Input: part model. Units: mm. Frame: model coordinates. A direction names the side the tool comes from. Round coordinates to 2 decimals unless told otherwise and drop trailing zeros. Loops run counter-clockwise (first coordinate to the right, second up) from the corner with the lowest first, then second, coordinate; pieces in that order, holes last.
1) First-contact query: pin 1 (3 mm diameter, centred on x = -9.5, y = 14, fed in from +Z); pin 2 (3 mm diameter, centred on x = -83.5, z = -66.5, fed in from -Y); pin 3 (4 mm diameter, centred on x = -109.51, z = 1.14, fed in from +Y). Flat tips, straight axial feed; report the tip coordinate or a pass-through.
2) Section B-B, the plane y = 12. Return loops of the section in (x, z) (3 decimals).
3) Section D-D, the plane x = -33.5. Return loops of the section in (y, z), and give its area (3 significant figures).
4) Section C-C, the plane z = -24. Return loops of the section in (x, y).
5) Section A-A, the plane y = 35.5. Return loops of the section in (x, z), and give its area (3 significant figures).
6) Ray query, line 1 along Z through (x, y) = (-47, 4); line 2 along X through (y, z) = (34.5, -31); line 3 along X through (y, z) = (33, -42.5). Return the intervals inside material, ascending.
7) Draft query along Z for faces 1 (the face through (-37.63, 34.53, -57.46)), 2 (the face through (-104.37, 18.68, -4.43)), 3 (the face through (-7, 32.675, -104)). Return one class per face: pulls with the +Z half, pulls with the -Z half, needs draft (parallel to the pull), parting line crosses it, or undercut.
8) Access query for faces 4 (the face through (-103.37, 3.13, -86.91)), 5 (the face through (-107, 32.675, 0)), 6 (the face through (-103.944, 18.682, -98.721)), 7 (the face through (-7, 32.675, -1)). Directions: +Z, -Z, +X, -X, +Y, -Y. A direction counts if a zero-diameter tool reaches every point of the face in a straight line with its end or side. Return the directions, or none.
from build123d import *

# Parameters (mm, degrees)
SKETCH1_W           = 119.38
SKETCH1_H           = 119.38
BOSS_EXTRUDE1_DEPTH = 37.75
SKETCH2_R           = 2.286
CUT_EXTRUDE1_DEPTH  = 38.75
SKETCH3_R           = 58.41973455
CUT_EXTRUDE2_DEPTH  = 6.35
SKETCH4_R           = 58.42
CUT_EXTRUDE3_DEPTH  = 6.35
SKETCH5_R           = 20.32
BOSS_EXTRUDE2_DEPTH = 6.35
SKETCH6_R           = 20.32
BOSS_EXTRUDE3_DEPTH = 6.35
FILLET1_R           = 5.08
SKETCH7_R           = 88.9
SKETCH7_R_2         = 66.675
CUT_EXTRUDE5_DEPTH  = 13.8


with BuildPart() as part:
    # Sketch1 → Boss-Extrude1 (new body)
    with BuildSketch(Plane(origin=(0, 0, 0), x_dir=(1, 0, 0), z_dir=(0, 1, 0))):
        with Locations((-57.011822664, 51.361162791)):
            Rectangle(SKETCH1_W, SKETCH1_H)
    extrude(amount=BOSS_EXTRUDE1_DEPTH)

    # Sketch2 → Cut-Extrude1 (cut, through all)
    with BuildSketch(Plane(origin=(0, 37.75, 0), x_dir=(1, 0, 0), z_dir=(0, 1, 0))):
        with Locations((-109.511822664, 103.861162791)):
            Circle(SKETCH2_R)
        with Locations((-4.511822664, 103.861162791)):
            Circle(SKETCH2_R)
        with Locations((-4.511822664, -1.138837209)):
            Circle(SKETCH2_R)
        with Locations((-109.511822664, -1.138837209)):
            Circle(SKETCH2_R)
    extrude(amount=-CUT_EXTRUDE1_DEPTH, mode=Mode.SUBTRACT)

    # Sketch3 → Cut-Extrude2 (cut)
    with BuildSketch(Plane(origin=(0, 37.75, 0), x_dir=(1, 0, 0), z_dir=(0, 1, 0))):
        with Locations((-57.011822664, 51.361162791)):
            Circle(SKETCH3_R)
    extrude(amount=-CUT_EXTRUDE2_DEPTH, mode=Mode.SUBTRACT)

    # Sketch4 → Cut-Extrude3 (cut)
    with BuildSketch(Plane.XZ):
        with Locations((-57.011822664, -51.361162791)):
            Circle(SKETCH4_R)
    extrude(amount=-CUT_EXTRUDE3_DEPTH, mode=Mode.SUBTRACT)

    # Sketch5 → Boss-Extrude2 (add)
    with BuildSketch(Plane.XZ.offset(-6.35)):
        with Locations((-57.011822664, -51.361162791)):
            Circle(SKETCH5_R)
    extrude(amount=BOSS_EXTRUDE2_DEPTH)

    # Sketch6 → Boss-Extrude3 (add)
    with BuildSketch(Plane(origin=(0, 31.4, 0), x_dir=(1, 0, 0), z_dir=(0, 1, 0))):
        with Locations((-57.011822664, 51.361162791)):
            Circle(SKETCH6_R)
    extrude(amount=BOSS_EXTRUDE3_DEPTH)

    # Fillet1
    fillet1_edges = [part.edges().sort_by_distance(p)[0] for p in [
        (2.678177336, 18.875, 8.328837209),
        (-116.701822664, 18.875, 8.328837209),
        (-116.701822664, 18.875, -111.051162791),
        (2.678177336, 18.875, -111.051162791),
    ]]
    fillet(fillet1_edges, radius=FILLET1_R)

    # Sketch7 → Cut-Extrude5 (cut, symmetric)
    with BuildSketch(Plane(origin=(0, 18.875, 0), x_dir=(1, 0, 0), z_dir=(0, 1, 0))):
        with Locations((-57.011822664, 51.361162791)):
            Circle(SKETCH7_R)
        with Locations((-57.011822664, 51.361162791)):
            Circle(SKETCH7_R_2, mode=Mode.SUBTRACT)
    extrude(amount=CUT_EXTRUDE5_DEPTH, both=True, mode=Mode.SUBTRACT)


solid = part.part
Final values:
1. pin 1: stops at z = -3.11
1. pin 2: stops at y = 6.35
1. pin 3: passes through
2. outline: (-116.702, -81.071) arc R66.675 ccw to (-86.721, -111.051) - (-27.302, -111.051) arc R66.675 ccw to (2.678, -81.071) - (2.678, -21.652) arc R66.675 ccw to (-27.302, 8.329) - (-86.721, 8.329) arc R66.675 ccw to (-116.702, -21.652) - close
3. outline: (0, -111.05) - (37.75, -111.05) - (37.75, -104.84) - (31.4, -104.84) - (31.4, 2.12) - (37.75, 2.12) - (37.75, 8.33) - (0, 8.33) - (0, 2.12) - (6.35, 2.12) - (6.35, -104.84) - (0, -104.84) - close
3. area: 3,150 mm2
4. outline: (-116.7, 0) - (-108.63, 0) - (-108.63, 6.35) - (-5.4, 6.35) - (-5.4, 0) - (2.68, 0) - (2.68, 37.75) - (-5.4, 37.75) - (-5.4, 31.4) - (-108.63, 31.4) - (-108.63, 37.75) - (-116.7, 37.75) - close
5. outline: (-116.7, -105.97) arc R5.08 ccw to (-111.62, -111.05) - (-2.4, -111.05) arc R5.08 ccw to (2.68, -105.97) - (2.68, 3.25) arc R5.08 ccw to (-2.4, 8.33) - (-111.62, 8.33) arc R5.08 ccw to (-116.7, 3.25) - close; circle Ø40.64 at (-57.01, -51.36); hole circle Ø116.84 at (-57.01, -51.36); hole circle Ø4.57 at (-109.51, -103.86); hole circle Ø4.57 at (-109.51, 1.14); hole circle Ø4.57 at (-4.51, -103.86); hole circle Ø4.57 at (-4.51, 1.14)
5. area: 4,740 mm2
6. line 1: z = -111.05 to -108.92, -69.04 to -33.68, 6.19 to 8.33
6. line 2: x = -116.7 to -111.77, -2.26 to 2.68
6. line 3: x = -116.7 to -114.76, -75.3 to -38.73, 0.73 to 2.68
7. face 1: undercut
7. face 2: pulls with the +Z half
7. face 3: needs draft
8. face 4: -Y
8. face 5: +Z, -X
8. face 6: -Z, -X
8. face 7: +Z, +X
